CAD build for the part. Positions are in the model's coordinates, mm. A direction names the side the tool comes from. Coordinates: 2 decimals unless noted, no trailing zeros. Write each loop counter-clockwise with the first axis right and the second up, starting at its lowest first coordinate (ties: lowest second). Pieces come first, ordered by that corner, then holes. Notation, with made-up numbers: M 61,4 L 98,4 A17 cw 98,11 Z; hole C 68.25,-31 d4. An arc over 180 degrees is marked long. Answer as CSV lines item,"result". Start each with the question number.
```python
from build123d import *

# Parameters (mm, degrees)
BOSS_EXTRUDE2_DEPTH = 40
CUT_EXTRUDE6_DEPTH  = 20
SKETCH11_R          = 15
BOSS_EXTRUDE3_DEPTH = 80
CUT_EXTRUDE7_DEPTH  = 20
CUT_EXTRUDE9_START  = -20
CUT_EXTRUDE9_DEPTH  = 20
SKETCH15_R          = 15
CUT_EXTRUDE10_DEPTH = 40


with BuildPart() as part:
    # Sketch4 → Boss-Extrude2 (new, symmetric)
    with BuildSketch(Plane.XY):
        with BuildLine():
            Line((-250, 50), (250, 50))
            ThreePointArc((250, 50), (300, 0), (250, -50))
            Line((250, -50), (-250, -50))
            ThreePointArc((-250, -50), (-300, 0), (-250, 50))
        make_face()
    extrude(amount=BOSS_EXTRUDE2_DEPTH, both=True)

    # Sketch10 → Cut-Extrude6 (cut, symmetric)
    with BuildSketch(Plane.XY):
        with BuildLine():
            Line((150, 50), (250, 50))
            ThreePointArc((250, 50), (300, 0), (250, -50))
            Line((250, -50), (150, -50))
            ThreePointArc((150, -50), (200, 0), (150, 50))
        make_face()
    extrude(amount=CUT_EXTRUDE6_DEPTH, both=True, mode=Mode.SUBTRACT)

    # Sketch11 → Boss-Extrude3 (add)
    with BuildSketch(Plane.XY.offset(40)):
        with Locations((250, 0)):
            Circle(SKETCH11_R)
    extrude(amount=-BOSS_EXTRUDE3_DEPTH)

    # Sketch12 → Cut-Extrude7 (cut)
    with BuildSketch(Plane.XY.offset(40)):
        with BuildLine():
            Line((250, 50), (73.543550677, 14.708710135))
            ThreePointArc((73.543550677, 14.708710135), (61.485292704, 0), (73.543550677, -14.708710135))
            Line((73.543550677, -14.708710135), (250, -50))
            Line((250, -50), (-250, -50))
            ThreePointArc((-250, -50), (-300, 0), (-250, 50))
            Line((-250, 50), (250, 50))
        make_face()
    extrude(amount=-CUT_EXTRUDE7_DEPTH, mode=Mode.SUBTRACT)

    # Sketch14 → Cut-Extrude9 (cut)
    with BuildSketch(Plane(origin=(0, 0, -40), x_dir=(-1, 0, 0), z_dir=(0, 0, -1)).offset(CUT_EXTRUDE9_START)):
        with BuildLine():
            Line((-73.543550677, -14.708710135), (-250, -50))
            Line((-250, -50), (250, -50))
            ThreePointArc((250, -50), (300, 0), (250, 50))
            Line((250, 50), (-250, 50))
            Line((-250, 50), (-73.543550677, 14.708710135))
            ThreePointArc((-73.543550677, 14.708710135), (-61.485292704, 0), (-73.543550677, -14.708710135))
        make_face()
    extrude(amount=CUT_EXTRUDE9_DEPTH, mode=Mode.SUBTRACT)

    # Sketch15 → Cut-Extrude10 (cut)
    with BuildSketch(Plane(origin=(0, 0, -20), x_dir=(-1, 0, 0), z_dir=(0, 0, -1))):
        with Locations((250, 0)):
            Circle(SKETCH15_R)
    extrude(amount=-CUT_EXTRUDE10_DEPTH, mode=Mode.SUBTRACT)


with BuildPart() as part_1:
    # Body-Move/Copy1: moved
    add(part.part.moved(Location((250, 0, 0))))


solid = part_1.part
```
1) Pin check, flat tips, straight feed: P1, Ø2, axis at x = 174.5, y = 17, coming from the +Z side; P2, Ø12, axis at y = 32, z = -24, coming from the -X side; P3, Ø4, axis at x = 42, y = -12, coming from the -Z side; P4, Ø3, axis at x = 370.5, z = -20.5, coming from the -Y side. Stop position of each tip, or through.
2) Two-plate mould, pull along Z, no slides. Class faces 1 (the cylindrical face through (-13.856, -5.745, -0.28)), 2 (the flat face through (459, 1, -40)), 3 (the flat face through (480, 1, -20)), 4 (the cylindrical face through (513.856, -5.745, 0.28)): pulls with the +Z half, pulls with the -Z half, needs draft (parallel to the pull), parting line crosses it, or undercut.
3) Band-saw the part on B-B, the plane z = -10.5. List the corners of the cut face in (x, y), plus the area to 3 significant figures.
4) Tool access for faces 5 (the flat face through (410.5, -32.1, 30.1)), 6 (the cylindrical face through (311.49, 0.29, 30.14)), 7 (the cylindrical face through (311.49, 0.29, -29.86)), 8 (the flat face through (410.5, -32.1, -29.9)), 9 (the flat face through (413, 32.6, -29.9)): list every direction of +Z, -Z, +X, -X, +Y, -Y with a clear straight run to the whole face (end or side of a thin tool).
5) Probe L1, parallel to Z at x = 486, y = 14; L2, parallel to Y at x = 0, z = 10; L3, parallel to Z at x = 108.5, y = -40. List the from-to ranges inside material, lowest first. Write a range as [from, to].
6) Band-saw the part on A-A, the plane y = 0. List the corners of the cut face in (x, z), plus the area to 3 significant figures.
7) Band-saw the part on D-D, the plane y = -31. List the corners of the cut face in (x, z), plus the area to 3 significant figures.
8) Band-saw the part on C-C, the plane x = 42. List the corners of the cut face in (y, z).
Result sheet:
1,P1,"stops at z = 20"
1,P2,"stops at x = -41.74"
1,P3,"stops at z = -20"
1,P4,"stops at y = -50"
2,face 1,"needs draft"
2,face 2,"pulls with the -Z half"
2,face 3,"undercut"
2,face 4,"undercut"
3,outline,"M 0,-50 L 400,-50 A50 ccw 400,50 L 0,50 A50 ccw Z; C 500,0 d30; hole C 0,0 d30"
3,area,"47,900 mm²"
4,face 5,"+Z, -X, -Y"
4,face 6,"+Z, -X"
4,face 7,"-Z, -X"
4,face 8,"-Z, -X, -Y"
4,face 9,"-Z, -X, +Y"
5,L1,"z = [-40, -20], [20, 40]"
5,L2,"y = [-50, -15], [15, 50]"
5,L3,"z = [-20, 20]"
6,outline,"M -50,-20 L -15,-20 L -15,20 L -50,20 Z; M 15,-20 L 311.49,-20 L 311.49,-40 L 550,-40 L 550,-20 L 515,-20 L 515,20 L 550,20 L 550,40 L 311.49,40 L 311.49,20 L 15,20 Z; hole M 450,-20 L 485,-20 L 485,20 L 450,20 Z"
6,area,"29,500 mm²"
7,outline,"M -39.23,-20 L 405,-20 L 405,-40 L 539.23,-40 L 539.23,-20 L 439.23,-20 L 439.23,20 L 539.23,20 L 539.23,40 L 405,40 L 405,20 L -39.23,20 Z"
7,area,"24,500 mm²"
8,outline,"M -50,-20 L 50,-20 L 50,20 L -50,20 Z"
